Geometry check sheet. Reference: the model listing, model coordinates, mm. A direction names the side the tool comes from. Give positions to 0.01 mm unless a question says otherwise; leave off trailing zeros. Order: outer loops, then holes, each group sorted by start corner. A loop starts at its lowest first (then second) coordinate and runs counter-clockwise, first axis right, second up. Notation, with made-up numbers: M 35.25,70 L 63.25,70 A16 ccw 63.25,98 Z; hole C 62.5,74.5 d2. An arc over 180 degrees is marked long. Answer as CSV lines item,"result". Start each with the question number.
Q1. Section check A-A, the plane x = -88. Record the boundary of the cut face in (y, z).
Q2. Go/stop test with flat-tipped pins: pin 1 (0.5 mm diameter, centred on x = -89.5, y = 0.5, fed in from -Z); pin 2 (3 mm diameter, centred on x = 0, z = 271.25, fed in from -Y); pin 3 (0.5 mm diameter, centred on x = 79, y = 0.5, fed in from +Z). Record where each tip stops, or that it passes through.
Q3. Section check B-B, the plane z = 187. Record the boundary of the cut face in (x, y), then the cut area to 3 significant figures.
Q4. Section check C-C, the plane x = 86. Record the boundary of the cut face in (y, z).
Q5. Thickness scan on line 1 (X direction, y = 0.35, z = 219); line 2 (X direction, y = 0.2, z = 251); line 3 (Z direction, x = 89, y = 0.9). Record the ranges inside material, lowest first.
Q6. Set-up check for faces 4 (the cylindrical face through (-42.36, 0.493, 93.086)), 5 (the flat face through (93.6, 0.5, 188.9)): record each of +Z, -Z, +X, -X, +Y, -Y from which the full face is reachable in a straight line by a thin tool's end or side.
Q7. Mould release check, pull along X, two halves, no side actions. Record for faces 1 (the flat face through (-58.554, 0.493, 250.41)), 2 (the cylindrical face through (42.92, 0.49, 92.95)), 3 (the flat face through (-1, 1, 4)): +X half, -X half, draft (parallel to the pull), parting line (faces both ways), or undercut.
Q8. Section check D-D, the plane y = 0.4. Count the separate pieces of the cut face and the enclosed holes in it, then the cut area to 3 significant figures.
```python
from build123d import *

# Parameters (mm, degrees)
SKETCH1_R           = 1.25
BOSS_EXTRUDE1_DEPTH = 1


with BuildPart() as part:
    # Sketch1 → Boss-Extrude1 (new body)
    with BuildSketch(Plane(origin=(0, 0, 0), x_dir=(1, 0, 0), z_dir=(0, 1, 0))):
        with BuildLine():
            Line((-35.214466094, -273.75), (35.214466094, -273.75))
            Line((35.214466094, -273.75), (81.25, -227.714466094))
            Line((81.25, -227.714466094), (81.25, -201.25))
            Line((81.25, -201.25), (106.25, -176.25))
            Line((106.25, -176.25), (106.25, -88.874002831))
            ThreePointArc((106.25, -88.874002831), (104.785533906, -85.338468925), (101.25, -83.874002831))
            Line((101.25, -83.874002831), (66.605380572, -83.874002831))
            ThreePointArc((66.605380572, -83.874002831), (63.947538367, -84.23367738), (61.480887801, -85.286827869))
            ThreePointArc((61.480887801, -85.286827869), (42.637913048, -93.018246989), (22.356633062, -94.889669244))
            ThreePointArc((22.356633062, -94.889669244), (18.9756934, -93.299812922), (17.640548545, -89.810431267))
            Line((17.640548545, -89.810431267), (17.793393264, -81.053963175))
            ThreePointArc((17.793393264, -81.053963175), (19.401963586, -77.466532095), (23.106937946, -76.151113824))
            ThreePointArc((23.106937946, -76.151113824), (38.512493282, -74.722995147), (52.743936183, -68.653671368))
            ThreePointArc((52.743936183, -68.653671368), (55.286579623, -67.521722803), (58.04272342, -67.134405642))
            Line((58.04272342, -67.134405642), (101.25, -67.134405642))
            ThreePointArc((101.25, -67.134405642), (104.785533906, -65.669939548), (106.25, -62.134405642))
            Line((106.25, -62.134405642), (106.25, 140.817393532))
            Line((106.25, 140.817393532), (63.754385783, 208.997474683))
            Line((63.754385783, 208.997474683), (63.754385783, 254.885164258))
            Line((63.754385783, 254.885164258), (58.833815977, 258.997474683))
            Line((58.833815977, 258.997474683), (-58.833815977, 258.997474683))
            Line((-58.833815977, 258.997474683), (-63.754385783, 254.885164258))
            Line((-63.754385783, 254.885164258), (-63.754385783, 208.997474683))
            Line((-63.754385783, 208.997474683), (-106.25, 140.817393532))
            Line((-106.25, 140.817393532), (-106.25, -62.134405642))
            ThreePointArc((-106.25, -62.134405642), (-104.785533906, -65.669939548), (-101.25, -67.134405642))
            Line((-101.25, -67.134405642), (-58.04272342, -67.134405642))
            ThreePointArc((-58.04272342, -67.134405642), (-55.286579623, -67.521722803), (-52.743936183, -68.653671368))
            ThreePointArc((-52.743936183, -68.653671368), (-38.512493282, -74.722995147), (-23.106937946, -76.151113824))
            ThreePointArc((-23.106937946, -76.151113824), (-19.401963586, -77.466532095), (-17.793393264, -81.053963175))
            Line((-17.793393264, -81.053963175), (-17.640548545, -89.810431267))
            ThreePointArc((-17.640548545, -89.810431267), (-18.9756934, -93.299812922), (-22.356633062, -94.889669244))
            ThreePointArc((-22.356633062, -94.889669244), (-42.637913048, -93.018246989), (-61.480887801, -85.286827869))
            ThreePointArc((-61.480887801, -85.286827869), (-63.947538367, -84.23367738), (-66.605380572, -83.874002831))
            Line((-66.605380572, -83.874002831), (-101.25, -83.874002831))
            ThreePointArc((-101.25, -83.874002831), (-104.785533906, -85.338468925), (-106.25, -88.874002831))
            Line((-106.25, -88.874002831), (-106.25, -176.25))
            Line((-106.25, -176.25), (-81.25, -201.25))
            Line((-81.25, -201.25), (-81.25, -227.714466094))
            Line((-81.25, -227.714466094), (-35.214466094, -273.75))
        make_face()
        with Locations(Location((0, 256.50465463, 0), (0, 0, 270))):
            Circle(SKETCH1_R, mode=Mode.SUBTRACT)
        with Locations(Location((-102.8125, -50.9375, 0), (0, 0, 270))):
            Circle(SKETCH1_R, mode=Mode.SUBTRACT)
        with Locations(Location((0, -50, 0), (0, 0, 270))):
            Circle(SKETCH1_R, mode=Mode.SUBTRACT)
        with Locations(Location((0, -271.25, 0), (0, 0, 270))):
            Circle(SKETCH1_R, mode=Mode.SUBTRACT)
        with Locations(Location((102.8125, -50.9375, 0), (0, 0, 90))):
            Circle(SKETCH1_R, mode=Mode.SUBTRACT)
    extrude(amount=BOSS_EXTRUDE1_DEPTH)


solid = part.part
```
Answer block:
1,outline,"M 0,-170.1 L 1,-170.1 L 1,67.13 L 0,67.13 Z; M 0,83.87 L 1,83.87 L 1,194.5 L 0,194.5 Z"
2,pin 1,"stops at z = -168.09"
2,pin 2,"stops at y = 0"
2,pin 3,"stops at z = 230.21"
3,outline,"M -95.5,0 L 95.5,0 L 95.5,1 L -95.5,1 Z"
3,area,"191 mm2"
4,outline,"M 0,-173.31 L 1,-173.31 L 1,67.13 L 0,67.13 Z; M 0,83.87 L 1,83.87 L 1,196.5 L 0,196.5 Z"
5,line 1,"x = -81.25 to 81.25"
5,line 2,"x = -57.96 to 57.96"
5,line 3,"z = -168.49 to 67.13, 83.87 to 193.5"
6,face 4,"+Y, -Y"
6,face 5,"+Z, +X, +Y, -Y"
7,face 1,"-X half"
7,face 2,"undercut"
7,face 3,"draft"
8,separate pieces,"1"
8,enclosed holes,"5"
8,area,"96,400 mm2"
